Geometry check sheet. Reference: drawing and pictorial views, mm from the part's lowest x, y, z. Give positions to 0.01 mm unless a question says otherwise; leave off trailing zeros. Write each question's results on one line, items separated by ' | '. Start each with the question number.
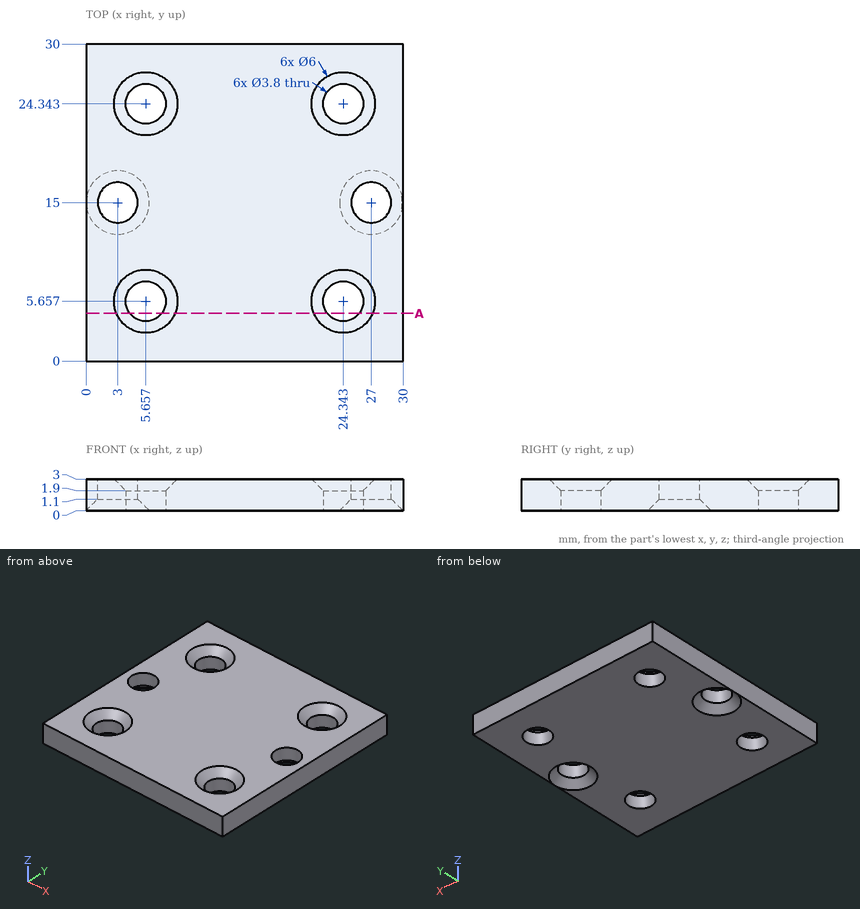
Q1. Section check A-A on y = 4.5. State how many separate pieces and enclosed holes the cut face has, plus the area to 3 significant figures.
Q2. Scan lines: L1, parallel to Y at x = 5.5, z = 2.25; L2, parallel to X at y = 16, z = 0.45 (1 decimal); L3, parallel to X at y = 4, z = 2.8 (1 decimal). Record each from-to range of solid material in increasing order.
Q3. Depth check by flat-ended pin: pin 1 Ø5 at (x, y) = (5.66, 5.66) entering from -Z; pin 2 Ø3 at (x, y) = (24.34, 5.66) entering from +Z; pin 3 Ø4.5 at (x, y) = (24.34, 24.34) entering from +Z (1 decimal). Enter the tip coordinate at first touch or a pass-through.
Check result:
1) separate pieces: 3 | enclosed holes: 0 | area: 69.1 mm^2
2) L1: 0 to 3.41, 7.9 to 22.1, 26.59 to 30 | L2: 0 to 0.7, 5.3 to 24.7, 29.3 to 30 | L3: 0 to 3.4, 7.9 to 22.1, 26.6 to 30
3) pin 1: z = 0 | pin 2: through | pin 3: z = 2.3
